```python
from build123d import *

# Parameters (mm, degrees)
F0_W     = 10
F0_H     = 12
F1_DEPTH = 20
F2_W     = 2.8
F2_H     = 16
F3_DEPTH = 9.5
F4_SIZE  = 8
F5_SIZE  = 3
F6_R     = 2


with BuildPart() as f1:
    # F0 (on Front) → F1 (new body, symmetric)
    with BuildSketch(Plane.XZ):
        Rectangle(F0_W, F0_H)
    extrude(amount=F1_DEPTH, both=True)

    # F2 (on face) → F3 (cut)
    with BuildSketch(Plane(origin=(0, 0, -6), x_dir=(1, 0, 0), z_dir=(0, 0, -1))):
        Rectangle(F2_W, F2_H)
    extrude(amount=-F3_DEPTH, mode=Mode.SUBTRACT)

    # F4
    f4_edges = [f1.edges().sort_by_distance(p)[0] for p in [
        (0, -20, 6),
        (0, 20, 6),
    ]]
    chamfer(f4_edges, length=F4_SIZE)

    # F5
    f5_edges = [f1.edges().sort_by_distance(p)[0] for p in [
        (0, -12, 6),
        (0, 12, 6),
    ]]
    chamfer(f5_edges, length=F5_SIZE)

    # F6
    f6_edges = [f1.edges().sort_by_distance(p)[0] for p in [
        (5, 17.06066, 0.93934),
        (5, 11.56066, 4.93934),
        (5, 20, -4),
        (5, 0, 6),
        (5, 0, -6),
        (5, -11.56066, 4.93934),
        (5, -20, -4),
        (5, -17.06066, 0.93934),
        (-5, 0, 6),
        (-5, 11.56066, 4.93934),
        (-5, -11.56066, 4.93934),
        (-5, 17.06066, 0.93934),
        (-5, -17.06066, 0.93934),
        (-5, 20, -4),
        (-5, -20, -4),
        (-5, 0, -6),
        (0, -20, -6),
        (0, 20, -6),
        (0, 20, -2),
        (0, 14.12132, 3.87868),
        (0, 9, 6),
        (0, -9, 6),
        (0, -14.12132, 3.87868),
        (0, -20, -2),
    ]]
    fillet(f6_edges, radius=F6_R)


solid = f1.part
```
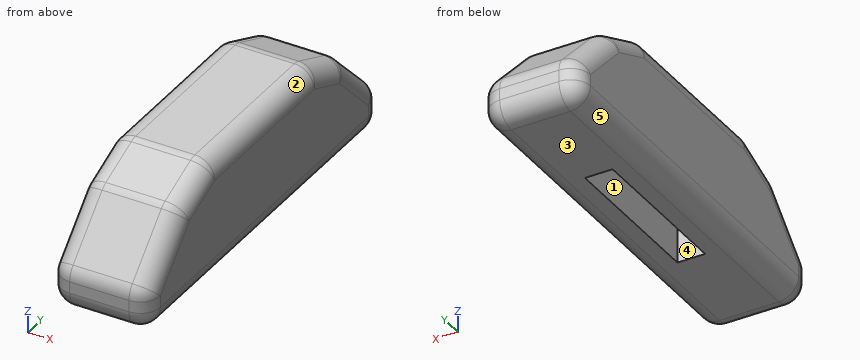
Source: CAD feature listing. Evaluate the final solid. Frame: model axes, mm. Face numbers are marked on the shaded views. A direction names the side the tool comes from. Round coordinates to 2 decimals unless told otherwise and drop trailing zeros. Order: outer loops, then holes, each group sorted by start corner. A loop starts at its lowest first (then second) coordinate and runs counter-clockwise, first axis right, second up. Notation, with made-up numbers: (88, 13) -> (93, 13) arc R18 ccw to (93, 21) -> close; hole circle Ø1 at (83.25, 38). An arc over 180 degrees is marked (long way). One line per item, written item: value. Start each with the question number.
Q1. Access query for the marked faces 1 and 2. Directions: +Z, -Z, +X, -X, +Y, -Y. A direction counts if a zero-diameter tool reaches every point of the face in a straight line with its end or side. Return the directions, or none.
Q2. Section query D-D (x = 0.5). Return the cut outline in (y, z).
Q3. Section query C-C (x = -2). Return the cut outline in (y, z), plus the area to 3 significant figures.
Q4. Pin query (flat end, axial travel): pin 1 (3 mm diameter, centred on x = 0.5, z = 1, fed in from -Y); pin 2 (2 mm diameter, centred on x = -0.5, z = 0.5, fed in from +Y). Return the tip coordinate at first contact, or that it passes through.
Q5. Material intervals for probe 1 along X at (y, z) = (-4.5, -0.5); probe 2 along Y at (x, z) = (-0.5, -4); probe 3 along Z at (x, y) = (1.25, 5.5), sorted ascending.
Q6. Draft query along X for the marked faces 3, 4 and 5. Return one class per face: pulls with the +X half, pulls with the -X half, needs draft (parallel to the pull), parting line crosses it, or undercut.
Q7. Section query B-B (y = -4.5). Return the cut outline in (x, z).
Q8. Section query A-A (z = -3.5). Return the cut outline in (x, y), plus the area to 3 significant figures.
Findings below:
1. face 1: -Z
1. face 2: +Z, +X, +Y, -Y
2. outline: (-20, -4) arc R2 ccw to (-18, -6) -> (-8, -6) -> (-8, 3.5) -> (8, 3.5) -> (8, -6) -> (18, -6) arc R2 ccw to (20, -4) -> (20, -2.83) arc R2 ccw to (19.41, -1.41) -> (14.4, 3.6) arc R2 ccw to (13.75, 4.03) -> (9.37, 5.85) arc R2 ccw to (8.6, 6) -> (-8.6, 6) arc R2 ccw to (-9.37, 5.85) -> (-13.75, 4.03) arc R2 ccw to (-14.4, 3.6) -> (-19.41, -1.41) arc R2 ccw to (-20, -2.83) -> close
3. outline: (-20, -4) arc R2 ccw to (-18, -6) -> (18, -6) arc R2 ccw to (20, -4) -> (20, -2.83) arc R2 ccw to (19.41, -1.41) -> (14.4, 3.6) arc R2 ccw to (13.75, 4.03) -> (9.37, 5.85) arc R2 ccw to (8.6, 6) -> (-8.6, 6) arc R2 ccw to (-9.37, 5.85) -> (-13.75, 4.03) arc R2 ccw to (-14.4, 3.6) -> (-19.41, -1.41) arc R2 ccw to (-20, -2.83) -> close
3. area: 408 mm²
4. pin 1: y = -18.5
4. pin 2: y = 18.5
5. probe 1: -5 to -1.4, 1.4 to 5
5. probe 2: -20 to -8, 8 to 20
5. probe 3: 3.5 to 6
6. face 3: needs draft
6. face 4: undercut
6. face 5: pulls with the -X half
7. outline: (-5, -4) arc R2 ccw to (-3, -6) -> (-1.4, -6) -> (-1.4, 3.5) -> (1.4, 3.5) -> (1.4, -6) -> (3, -6) arc R2 ccw to (5, -4) -> (5, 4) arc R2 ccw to (3, 6) -> (-3, 6) arc R2 ccw to (-5, 4) -> close
8. outline: (-5, -18) arc R2 ccw to (-3, -20) -> (3, -20) arc R2 ccw to (5, -18) -> (5, 18) arc R2 ccw to (3, 20) -> (-3, 20) arc R2 ccw to (-5, 18) -> close; hole (-1.4, -8) -> (1.4, -8) -> (1.4, 8) -> (-1.4, 8) -> close
8. area: 352 mm²
